from build123d import *

# Parameters (mm, degrees)
SKETCH_1_R            = 6
EXTRUDE_1_DEPTH       = 9.9
SKETCH_2_R            = 4.25
EXTRUDE_2_DEPTH       = 10.3
SKETCH_2_2_R          = 4.25
SKETCH_2_2_R_2        = 3.25
CUT_EXTRUDE_1_DEPTH   = 5
EXTRUDE_START         = 12.9
SKETCH_3_R            = 6.5
SKETCH_3_R_2          = 6
SKETCH_3_W            = 7.396157214
SKETCH_3_H            = 7.5
EXTRUDE_3_DEPTH       = 12.9
SKETCH_4_W            = 4.733909146
SKETCH_4_H            = 7.574967903
CUT_EXTRUDE_1_2_DEPTH = 12.9


with BuildPart() as part:
    # Sketch 1 → Extrude 1 (new body)
    with BuildSketch(Plane(origin=(0, 0, 0), x_dir=(1, 0, 0), z_dir=(0, 1, 0))):
        with Locations(Location((0, 0, 0), (0, 0, 90))):
            Circle(SKETCH_1_R)
    extrude(amount=EXTRUDE_1_DEPTH)

    # Sketch 2 → Extrude 2 (add)
    with BuildSketch(Plane(origin=(0, 9.9, 0), x_dir=(1, 0, 0), z_dir=(0, 1, 0))):
        with Locations(Location((0, 0, 0), (0, 0, 90))):
            Circle(SKETCH_2_R)
    extrude(amount=EXTRUDE_2_DEPTH)

    # Sketch 2_2 → Cut-Extrude 1 (cut)
    with BuildSketch(Plane(origin=(0, 9.9, 0), x_dir=(1, 0, 0), z_dir=(0, 1, 0))):
        Circle(SKETCH_2_2_R)
        Circle(SKETCH_2_2_R_2, mode=Mode.SUBTRACT)
    extrude(amount=CUT_EXTRUDE_1_DEPTH, mode=Mode.SUBTRACT)

    # Sketch 3 → Extrude 3 (add)
    with BuildSketch(Plane.XZ.offset(EXTRUDE_START)):
        with BuildLine():
            ThreePointArc((5.963205412, 0.663461538), (6.364386662, 1.929173588), (6.5, 3.25))
            Line((6.5, 3.25), (5.04356025, 3.25))
            ThreePointArc((5.04356025, 3.25), (5.653297081, 2.010032863), (5.963205412, 0.663461538))
        make_face()
        with BuildLine():
            Line((5.04356025, 3.25), (6.5, 3.25))
            ThreePointArc((6.5, 3.25), (0, 9.75), (-6.5, 3.25))
            Line((-6.5, 3.25), (-5.04356025, 3.25))
            ThreePointArc((-5.04356025, 3.25), (0, 6), (5.04356025, 3.25))
        make_face()
        with BuildLine():
            ThreePointArc((5.963205412, 0.663461538), (5.653297081, 2.010032863), (5.04356025, 3.25))
            Line((5.04356025, 3.25), (-5.04356025, 3.25))
            ThreePointArc((-5.04356025, 3.25), (-5.653297081, 2.010032863), (-5.963205412, 0.663461538))
            ThreePointArc((-5.963205412, 0.663461538), (0, -3.25), (5.963205412, 0.663461538))
        make_face()
        with BuildLine():
            Line((-5.04356025, 3.25), (-6.5, 3.25))
            ThreePointArc((-6.5, 3.25), (-6.364386662, 1.929173588), (-5.963205412, 0.663461538))
            ThreePointArc((-5.963205412, 0.663461538), (-5.653297081, 2.010032863), (-5.04356025, 3.25))
        make_face()
        with BuildLine():
            Line((-5.04356025, 3.25), (5.04356025, 3.25))
            ThreePointArc((5.04356025, 3.25), (0, 6), (-5.04356025, 3.25))
        make_face()
        with Locations((0, 3.25)):
            Circle(SKETCH_3_R)
        with Locations(Location((0, 0, 0), (0, 0, 270))):
            Circle(SKETCH_3_R_2)
        with BuildLine():
            Line((6.5, -13.25), (6.5, 3.25))
            ThreePointArc((6.5, 3.25), (6.364386662, 1.929173588), (5.963205412, 0.663461538))
            ThreePointArc((5.963205412, 0.663461538), (5.990794291, 0.332240521), (6, 0))
            ThreePointArc((6, 0), (-0.332240521, -5.990794291), (-5.963205412, 0.663461538))
            ThreePointArc((-5.963205412, 0.663461538), (-6.364386662, 1.929173588), (-6.5, 3.25))
            Line((-6.5, 3.25), (-6.5, -13.25))
            Line((-6.5, -13.25), (-3.527984912, -13.25))
            Line((-3.527984912, -13.25), (3.868172302, -13.25))
            Line((3.868172302, -13.25), (6.5, -13.25))
        make_face()
        with Locations((0.170093695, -17)):
            Rectangle(SKETCH_3_W, SKETCH_3_H)
    extrude(amount=-EXTRUDE_3_DEPTH)

    # Sketch 4 → Cut-Extrude 1 2 (cut)
    with BuildSketch(Plane(origin=(0, 0, 0), x_dir=(1, 0, 0), z_dir=(0, 1, 0))):
        with Locations((0.208089462, 16.962516048)):
            Rectangle(SKETCH_4_W, SKETCH_4_H)
    extrude(amount=-CUT_EXTRUDE_1_2_DEPTH, mode=Mode.SUBTRACT)


solid = part.part
Here's how the part is built. I have some questions about the finished solid (model axes, mm). A direction names the side the tool comes from. Round coordinates to 2 decimals unless told otherwise and drop trailing zeros. Order: outer loops, then holes, each group sorted by start corner. A loop starts at its lowest first (then second) coordinate and runs counter-clockwise, first axis right, second up. Notation, with made-up numbers: M 35,-16.75 L 54,-16.75 A27 cw 54,12.25 Z; hole C 27,-27 d7. An arc over 180 degrees is marked long. One line per question, with ' | ' between items.
1) Imagine slicing it at C-C, the plane x = 0. Write out the boundary of the cut face in (y, z), plus the area to 3 significant figures.
Checked values:
outline: M -12.9,-13.18 L 0,-13.18 L 0,-6 L 9.9,-6 L 9.9,-3.25 L 14.9,-3.25 L 14.9,-4.25 L 20.2,-4.25 L 20.2,4.25 L 14.9,4.25 L 14.9,3.25 L 9.9,3.25 L 9.9,6 L 0,6 L 0,9.75 L -12.9,9.75 Z | area: 492 mm²
2) We'd pull the mould along Y, two halves only. Please class faces 1 (the flat face through (0, 0, -9)), 2 (the flat face through (3, 9.9, -3)), 3 (the flat face through (6.5, -7, -5)): released by +Y, released by -Y, zero draft, split by the parting line, or undercut.
Checked values:
face 1: released by +Y | face 2: undercut | face 3: zero draft
3) I'm going to push flat-ended pins straight in: pin 1 Ø4 at (x, y) = (-0.5, 13) entering from -Z; pin 2 Ø2 at (y, z) = (-4.5, -18.5) entering from +X; pin 3 Ø2.5 at (y, z) = (-3.5, -18) entering from -X. Where does each tip first touch, or does it pass through?
Checked values:
pin 1: stops at z = -4.25 | pin 2: stops at x = 3.87 | pin 3: stops at x = -3.53
4) On a 3-axis mill with a long thin cutter (end or side, diameter ignored), from which of +Z, -Z, +X, -X, +Y, -Y can I reach the whole of each face in a straight line? I mean faces 4 (the flat face through (-2.159, -6, -17)), 5 (the cylindrical face through (-1.802, 4.881, -5.723)), 6 (the flat face through (-5, -7, -13.25)), 7 (the flat face through (3.868, -7, -17)). Say none if no direction works.
Checked values:
face 4: -Z, +Y, -Y | face 5: +Y | face 6: -Z, -X, +Y, -Y | face 7: -Z, +X, +Y, -Y
5) Imagine slicing it at D-D, the plane z = 0. Write out the boundary of the cut face in (x, y).
Checked values:
outline: M -6.5,-12.9 L 6.5,-12.9 L 6.5,0 L 6,0 L 6,9.9 L 3.25,9.9 L 3.25,14.9 L 4.25,14.9 L 4.25,20.2 L -4.25,20.2 L -4.25,14.9 L -3.25,14.9 L -3.25,9.9 L -6,9.9 L -6,0 L -6.5,0 Z
6) Imagine slicing it at B-B, the plane y = -5. Write out the boundary of the cut face in (x, z).
Checked values:
outline: M -6.5,-13.25 L -3.53,-13.25 L -3.53,-20.75 L -2.16,-20.75 L -2.16,-13.18 L 2.58,-13.18 L 2.58,-20.75 L 3.87,-20.75 L 3.87,-13.25 L 6.5,-13.25 L 6.5,3.25 A6.5 ccw -6.5,3.25 Z
7) Imagine slicing it at A-A, the plane z = -16. Write out the boundary of the cut face in (x, y), plus the area to 3 significant figures.
Checked values:
outline: M -3.53,-12.9 L -2.16,-12.9 L -2.16,0 L -3.53,0 Z; M 2.58,-12.9 L 3.87,-12.9 L 3.87,0 L 2.58,0 Z | area: 34.3 mm²
8) I need wall thicknesses on line 1 (Y direction, x = -2.75, z = -2); line 2 (Y direction, x = 4, z = -3); line 3 (Y direction, x = -2.75, z = -10.5). Which ranges of each line are inside material? Lowest first, please.
Checked values:
line 1: y = -12.9 to 9.9, 14.9 to 20.2 | line 2: y = -12.9 to 9.9 | line 3: y = -12.9 to 0
